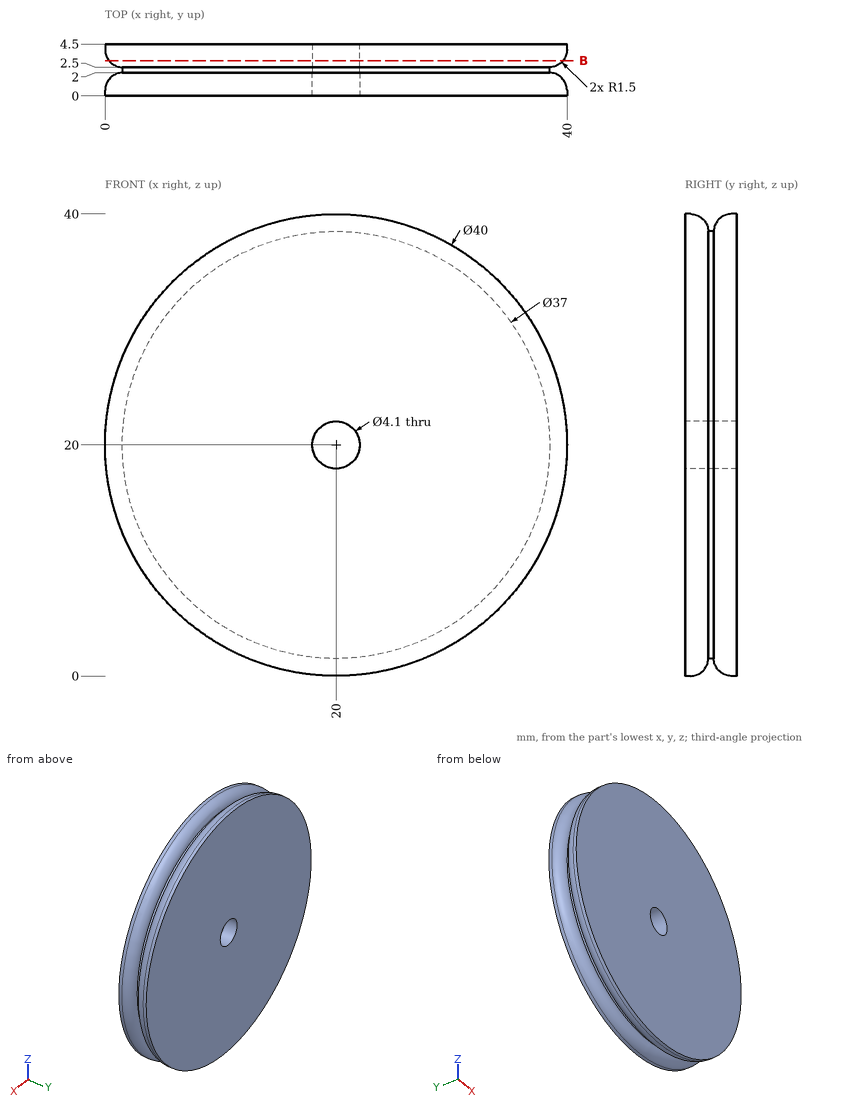
For this review, use the dimensioned drawing (mm, ordinates from the lowest corner) and the shaded views. Coordinates: 2 decimals unless noted, no trailing zeros. Write each loop counter-clockwise with the first axis right and the second up, starting at its lowest first coordinate (ties: lowest second). Pieces come first, ordered by that corner, then holes. Notation, with made-up numbers: (58, -36.75) -> (101, -36.75) arc R29 ccw to (101, -16.75) -> close; hole circle Ø5 at (14, -3.5). An arc over 180 degrees is marked (long way). Put each result on its own line as item: value.
Q1. Wall thickness on L1, parallel to Z at x = 20, y = 0.65; L2, parallel to Z at x = 20, y = 1.25: over which ranges is each line inside the solid? List them lowest first.
From the geometry:
L1: z = 0.01 to 17.95, 22.05 to 39.99
L2: z = 0.2 to 17.95, 22.05 to 39.8
Q2. Clearance check with a flat-ended pin moving along its axis: pin 1 Ø4.5 at (x, z) = (20, 20) entering from -Y. State where the tip first meets the part, or that it passes through.
From the geometry:
pin 1: stops at y = 0
Q3. Take a section at B-B, the plane y = 3.05. State the section outline as (x, z) points.
From the geometry:
outline: circle Ø39.32 at (20, 20); hole circle Ø4.1 at (20, 20)
